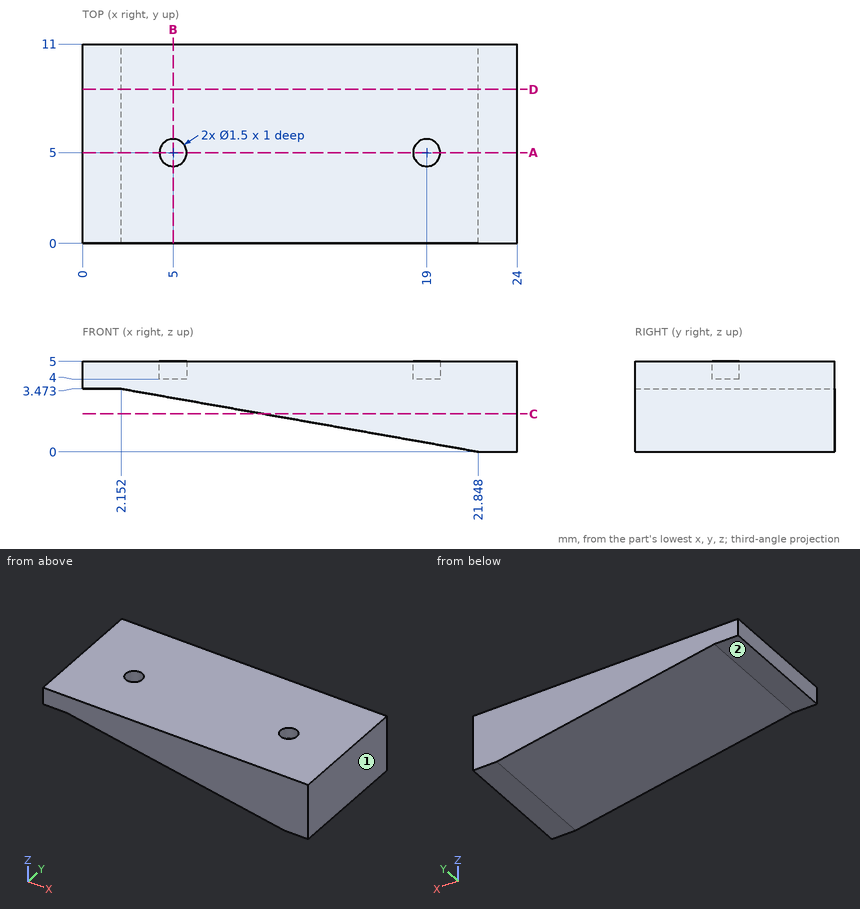
Answer from the drawing. Dimensions are ordinates in mm from the lowest x, y and z of the part. A direction names the side the tool comes from. Give positions to 0.01 mm unless a question says otherwise; leave off trailing zeros. Order: outer loops, then holes, each group sorted by start corner. A loop starts at its lowest first (then second) coordinate and runs counter-clockwise, first axis right, second up.
(1) Find section A-A (y = 5). Give the vertices of the cut face in (x, z), plus the area to 3 significant figures.
(2) For the marked faces 1 and 2, determine the directions among +Z, -Z, +X, -X, +Y, -Y from which every point of the face is accessible in a straight line to the end or side of a thin tool.
(3) Given pin 1 (6 mm diameter, centred on x = 11.5, y = 5.5, fed in from -Z); pin 2 (1.2 mm diameter, centred on x = 5, y = 5, fed in from -Z) (3 decimals); pin 3 (2 mm diameter, centred on x = 19, y = 5, fed in from -Z), each flat-ended and moving along its own axis, determine where each tip first touches the part or whether it passes through.
(4) Find section D-D (y = 8.5). Give the vertices of the cut face in (x, z), plus the area to 3 significant figures.
(5) Straight lines are drawn through the part: L1, parallel to Y at x = 5, z = 4.6; L2, parallel to Z at x = 2, y = 5.75; L3, parallel to Z at x = 19.75, y = 10.75. For each, find the intervals that lie inside material, in ascending order.
(6) Find section C-C (z = 2.1). Give the vertices of the cut face in (x, y).
(7) Find section B-B (x = 5). Give the vertices of the cut face in (y, z).
Result sheet:
1. outline: (0, 3.47) - (2.15, 3.47) - (21.85, 0) - (24, 0) - (24, 5) - (19.75, 5) - (19.75, 4) - (18.25, 4) - (18.25, 5) - (5.75, 5) - (5.75, 4) - (4.25, 4) - (4.25, 5) - (0, 5) - close
1. area: 75.3 mm2
2. face 1: +Z, -Z, +X, +Y, -Y
2. face 2: -Z, -X, +Y, -Y
3. pin 1: stops at z = 1.3
3. pin 2: stops at z = 2.865
3. pin 3: stops at z = 0.33
4. outline: (0, 3.47) - (2.15, 3.47) - (21.85, 0) - (24, 0) - (24, 5) - (0, 5) - close
4. area: 78.3 mm2
5. L1: y = 0 to 4.25, 5.75 to 11
5. L2: z = 3.47 to 5
5. L3: z = 0.37 to 5
6. outline: (9.94, 0) - (24, 0) - (24, 11) - (9.94, 11) - close
7. outline: (0, 2.97) - (11, 2.97) - (11, 5) - (5.75, 5) - (5.75, 4) - (4.25, 4) - (4.25, 5) - (0, 5) - close
